Work out the finished part from the listing and answer in its coordinate system (mm). A direction names the side the tool comes from. Round coordinates to 2 decimals unless told otherwise and drop trailing zeros. Loops run counter-clockwise (first coordinate to the right, second up) from the corner with the lowest first, then second, coordinate; pieces in that order, holes last.
```python
from build123d import *

# Parameters (mm, degrees)
SKETCH001_W     = 16.16
SKETCH001_H     = 16.16
SKETCH001_R     = 1.43
PAD_DEPTH       = 8
SKETCH002_W     = 10.16
SKETCH002_H     = 10.16
POCKET_DEPTH    = 5
SKETCH003_R     = 2.4
POCKET001_DEPTH = 3.081


with BuildPart() as part:
    # Sketch001 → Pad (new body)
    with BuildSketch(Plane.XY):
        with Locations((5, 5)):
            Rectangle(SKETCH001_W, SKETCH001_H)
        with Locations((2, 2)):
            Circle(SKETCH001_R, mode=Mode.SUBTRACT)
        with Locations((8, 2)):
            Circle(SKETCH001_R, mode=Mode.SUBTRACT)
    extrude(amount=PAD_DEPTH)

    # Sketch002 → Pocket (cut)
    with BuildSketch(Plane.XY.offset(8)):
        with Locations((5, 5)):
            Rectangle(SKETCH002_W, SKETCH002_H)
    extrude(amount=-POCKET_DEPTH, mode=Mode.SUBTRACT)

    # Sketch003 → Pocket001 (cut, through all)
    with BuildSketch(Plane.XZ.offset(-10)):
        with Locations((2.5, 9.5)):
            Circle(SKETCH003_R)
        with Locations((7.5, 9.5)):
            Circle(SKETCH003_R)
    extrude(amount=-POCKET001_DEPTH, mode=Mode.SUBTRACT)


solid = part.part
```
1. Which of the six approach directions +Z, -Z, +X, -X, +Y, -Y give full straight-line access (tool end or side, diameter ignored) to faces 1 (the face through (5, 10.08, 6)), 2 (the face through (7.5, 11.6, 7.1)), 3 (the face through (3.32, 1.45, 1.48))?
Answer key:
face 1: +Z
face 2: +Z, +Y
face 3: +Z, -Z
2. Consider probe 1 along Y at (x, z) = (8, 1.2); probe 2 along X at (y, z) = (2, 0.85); probe 3 along Y at (x, z) = (4, 6.25). Determine where each line is inside the solid, lowest interval first.
Answer key:
probe 1: y = -3.08 to 0.57, 3.43 to 13.08
probe 2: x = -3.08 to 0.57, 3.43 to 6.57, 9.43 to 13.08
probe 3: y = -3.08 to -0.08, 10.08 to 13.08
3. Determine the mould class of faces 4 (the face through (5, 12, 8)), 5 (the face through (5, 13.08, 4)), 6 (the face through (5, 5, 3)) for opening direction Y: +Y half, -Y half, draft (parallel to the pull), parting line (faces both ways), or undercut.
Answer key:
face 4: draft
face 5: +Y half
face 6: undercut
4. Find section A-A (y = 2). Write down the section's boundary in (x, z).
Answer key:
outline: (-3.08, 0) - (0.57, 0) - (0.57, 3) - (-0.08, 3) - (-0.08, 8) - (-3.08, 8) - close; (3.43, 0) - (6.57, 0) - (6.57, 3) - (3.43, 3) - close; (9.43, 0) - (13.08, 0) - (13.08, 8) - (10.08, 8) - (10.08, 3) - (9.43, 3) - close
5. Given pin 1 (4 mm diameter, centred on x = 6.5, y = 9, fed in from -Z); pin 2 (5 mm diameter, centred on x = 6, y = 6.5, fed in from +Z), each flat-ended and moving along its own axis, determine where each tip first touches the part or whether it passes through.
Answer key:
pin 1: stops at z = 0
pin 2: stops at z = 3
6. Find section C-C (x = 8.25). Write down the section's boundary in (y, z), then the cut area to 3 significant figures.
Answer key:
outline: (-3.08, 0) - (0.59, 0) - (0.59, 3) - (-0.08, 3) - (-0.08, 8) - (-3.08, 8) - close; (3.41, 0) - (13.08, 0) - (13.08, 7.22) - (10.08, 7.22) - (10.08, 3) - (3.41, 3) - close
area: 67.7 mm2
7. Find section D-D (z = 4). Write down the section's boundary in (x, y).
Answer key:
outline: (-3.08, -3.08) - (13.08, -3.08) - (13.08, 13.08) - (-3.08, 13.08) - close; hole (-0.08, -0.08) - (10.08, -0.08) - (10.08, 10.08) - (-0.08, 10.08) - close
8. Find section B-B (z = 0.5). Write down the section's boundary in (x, y), then the cut area to 3 significant figures.
Answer key:
outline: (-3.08, -3.08) - (13.08, -3.08) - (13.08, 13.08) - (-3.08, 13.08) - close; hole circle Ø2.86 at (2, 2); hole circle Ø2.86 at (8, 2)
area: 248 mm2
